Geometry check sheet. Reference: the model listing, model coordinates, mm. A direction names the side the tool comes from. Coordinates: 2 decimals unless noted, no trailing zeros. Loops run counter-clockwise (first coordinate to the right, second up) from the corner with the lowest first, then second, coordinate; pieces in that order, holes last. Notation, with made-up numbers: (-23, 27) - (15, 27) arc R23 cw to (15, 62) - close; hole circle Ø7 at (65.5, 54.5). An arc over 180 degrees is marked (long way). Write each question's results on one line, items separated by ' | '. Start each with the question number.
(1) Go/stop test with flat-tipped pins: pin 1 Ø4 at (y, z) = (-47.5, 82) entering from -X; pin 2 Ø12 at (x, y) = (103, -115.5) entering from -Z; pin 3 Ø8 at (x, y) = (-40, -109.5) entering from +Z; pin 4 Ø4 at (x, z) = (7.5, 45.5) entering from +Y. Record where each tip stops, or that it passes through.
(2) Sectioned sample at A-A (x = 34). Enter the section's corners in (y, z).
(3) Sectioned sample at B-B (z = 23). Enter the section's corners in (x, y).
(4) Mould release check, pull along Z, two halves, no side actions. Record for faces 1 (the face through (176, -93.98, 71)), 2 (the face through (175.386, -75, 32)), 3 (the face through (63, -76, 3.519)), 4 (the face through (-60, -47, 36.539)): pulls with the +Z half, pulls with the -Z half, needs draft (parallel to the pull), parting line crosses it, or undercut.
(5) Material ranges on probe 1 along Y at (x, z) = (3, 6.5); probe 2 along X at (y, z) = (-39, 20.5); probe 3 along Y at (x, z) = (140, 34.5), recorded low to high.
(6) Sectioned sample at D-D (x = 160.5). State how many separate pieces and enclosed holes the cut face has, plus the area to 3 significant figures.
(7) Sectioned sample at C-C (x = -23). Enter the section's corners in (y, z), plus the area to 3 significant figures.
(8) Access from +Z, -Z, +X, -X, +Y, -Y to the whole of each face (thin tool, end or side, straight path). Record for faces 5 (the face through (-53.214, -75, 32)), 6 (the face through (63, -50.8, 16)), 7 (the face through (176, -116.84, 71)).
from build123d import *

# Parameters (mm, degrees)
F0_W        = 254
F0_H        = 177.8
F1_DEPTH    = 152.4
F2_T        = -12.7
F3_T1_DEPTH = 342.9
F4_T1_DEPTH = 342.9
F5_W        = 22.86
F5_H        = 83.3190586418
F6_DEPTH    = 50.8
F7_W        = 22.86
F7_H        = 76.2
F8_DEPTH    = 50.8
F9_W        = 50.8
F9_H        = 25.4
F10_DEPTH   = 233.68
F11_W       = 254
F11_H       = 76.2
F12_DEPTH   = 180.34


# Not quite as in the source:
# - a fillet or chamfer that OpenCascade refuses, or shapes differently, is made with other operations: its cross-section is extruded or revolved along the edge and cut away or added


with BuildPart() as f1:
    # F0 (on Front) → F1 (new body)
    with BuildSketch(Plane.XZ):
        with Locations((61.0858832002, 0.9791328073)):
            Rectangle(F0_W, F0_H)
    extrude(amount=F1_DEPTH)

    # F2
    f2_openings = [f1.faces().sort_by_distance(p)[0] for p in [
        (61.085883, -76.2, -87.920867),
    ]]
    offset(amount=F2_T, openings=f2_openings)

    # F3: fillet of radius 38.1 on 1 edges, made by hand

    # F3_s2 → F3_t1 (cut)
    with BuildSketch(Plane.XZ.offset(-95.25)):
        with BuildLine():
            add(Edge.make_bspline(
                [(188.0858832002, 51.7791328073), (188.0858832002, 89.8791328073), (149.9858832002, 89.8791328073)],
                knots=[0, 0, 0, 1, 1, 1], degree=2, weights=[1, 1, 1]))
            Line((149.9858832002, 89.8791328073), (188.0858832002, 89.8791328073))
            Line((188.0858832002, 89.8791328073), (188.0858832002, 51.7791328073))
        make_face()
    extrude(amount=F3_T1_DEPTH, mode=Mode.SUBTRACT)

    # F4: fillet of radius 38.1 on 1 edges, made by hand

    # F4_s2 → F4_t1 (cut)
    with BuildSketch(Plane.XZ.offset(-95.25)):
        with BuildLine():
            add(Edge.make_bspline(
                [(-65.9141167998, 51.7791328073), (-65.9141167998, 89.8791328073), (-27.8141167998, 89.8791328073)],
                knots=[0, 0, 0, 1, 1, 1], degree=2, weights=[1, 1, 1]))
            Line((-27.8141167998, 89.8791328073), (-65.9141167998, 89.8791328073))
            Line((-65.9141167998, 89.8791328073), (-65.9141167998, 51.7791328073))
        make_face()
    extrude(amount=F4_T1_DEPTH, mode=Mode.SUBTRACT)

    # F5 (on face) → F6 (cut)
    with BuildSketch(Plane(origin=(-65.9141167998, 0, 0), x_dir=(0, -1, 0), z_dir=(-1, 0, 0))):
        with Locations((46.99, 78.1986621282)):
            Rectangle(F5_W, F5_H)
    extrude(amount=-F6_DEPTH, mode=Mode.SUBTRACT)

    # F7 (on face) → F8 (cut)
    with BuildSketch(Plane.YZ.offset(188.0858832002)):
        with Locations((-105.41, 74.6391328073)):
            Rectangle(F7_W, F7_H)
    extrude(amount=-F8_DEPTH, mode=Mode.SUBTRACT)

    # F9 (on face) → F10 (join)
    with BuildSketch(Plane(origin=(175.3858832002, 0, 0), x_dir=(0, -1, 0), z_dir=(-1, 0, 0))):
        with Locations((76.2, 16.2191328073)):
            Rectangle(F9_W, F9_H)
    extrude(amount=F10_DEPTH)

    # F11 (on face) → F12 (cut)
    with BuildSketch(Plane.XZ.offset(152.4)):
        with Locations((61.0858832002, -49.8208671927)):
            Rectangle(F11_W, F11_H)
    extrude(amount=-F12_DEPTH, mode=Mode.SUBTRACT)


solid = f1.part
Outcome:
1) pin 1: stops at x = -15.11 | pin 2: stops at z = 77.18 | pin 3: stops at z = 89.38 | pin 4: stops at y = 0
2) outline: (-152.4, -11.72) - (-139.7, -11.72) - (-139.7, 77.18) - (-12.7, 77.18) - (-12.7, -11.72) - (0, -11.72) - (0, 89.88) - (-152.4, 89.88) - close; (-101.6, 3.52) - (-50.8, 3.52) - (-50.8, 28.92) - (-101.6, 28.92) - close
3) outline: (-65.91, -152.4) - (188.09, -152.4) - (188.09, 0) - (-65.91, 0) - close; hole (-53.21, -139.7) - (175.39, -139.7) - (175.39, -101.6) - (-53.21, -101.6) - close; hole (-53.21, -50.8) - (175.39, -50.8) - (175.39, -12.7) - (-53.21, -12.7) - close
4) face 1: needs draft | face 2: undercut | face 3: pulls with the -Z half | face 4: pulls with the +Z half
5) probe 1: y = -152.4 to -139.7, -101.6 to -50.8, -12.7 to 0 | probe 2: x = -65.91 to -53.21, 175.39 to 188.09 | probe 3: y = -152.4 to -139.7, -12.7 to 0
6) separate pieces: 3 | enclosed holes: 0 | area: 5,080 mm2
7) outline: (-152.4, -11.72) - (-139.7, -11.72) - (-139.7, 77.18) - (-58.42, 77.18) - (-58.42, 89.88) - (-152.4, 89.88) - close; (-101.6, 3.52) - (-50.8, 3.52) - (-50.8, 28.92) - (-101.6, 28.92) - close; (-35.56, 77.18) - (-12.7, 77.18) - (-12.7, -11.72) - (0, -11.72) - (0, 89.88) - (-35.56, 89.88) - close | area: 5,190 mm2
8) face 5: none | face 6: -Z | face 7: +Z, +X
